Input: dimensioned drawing with shaded views. Units: mm. Origin: part minimum x, y, z. A direction names the side the tool comes from. Coordinates: 2 decimals unless noted, no trailing zeros. Write each loop counter-clockwise with the first axis right and the second up, starting at its lowest first coordinate (ties: lowest second). Pieces come first, ordered by that corner, then holes. Notation, with made-up numbers: (15.25, 8.5) -> (37.25, 8.5) arc R26 ccw to (37.25, 26.5) -> close; hole circle Ø5 at (-17, 63.5). An arc over 180 degrees is marked (long way). One line per item, written item: value. Start each with the question number.
1. Section query A-A, the plane y = 12. Output: boundary loops of the cut face in (x, z), and give its area (3 significant figures).
2. Access query for the marked faces 4 and 5. Directions: +Z, -Z, +X, -X, +Y, -Y. A direction counts if a zero-diameter tool reaches every point of the face in a straight line with its end or side. Return the directions, or none.
3. First-contact query: P1, Ø1.5, axis at x = 19, z = 3.5, coming from the +Y side; P2, Ø1, axis at y = 21, z = 3, coming from the -X side; P3, Ø7, axis at x = 12, y = 12, coming from the -Z side; P4, Ø8, axis at x = 11, y = 14.5, coming from the +Z side. Flat tips, straight axial feed; report the tip coordinate or a pass-through.
4. Mould query, pull axis X, two halves, no side actions, for the marked faces 1, 2 and 3. Classes: released by +X, released by -X, zero draft, split by the parting line, or undercut.
5. Section query D-D, the plane z = 4.6. Output: boundary loops of the cut face in (x, y).
6. Section query C-C, the plane z = 0.9. Output: boundary loops of the cut face in (x, y), and give its area (3 significant figures).
7. Line query: line 1 (Y direction, x = 12, z = 2.15); line 2 (Y direction, x = 12, z = 4.6); line 3 (Z direction, x = 17.5, y = 8.75). Output: solid intervals per line, ascending.
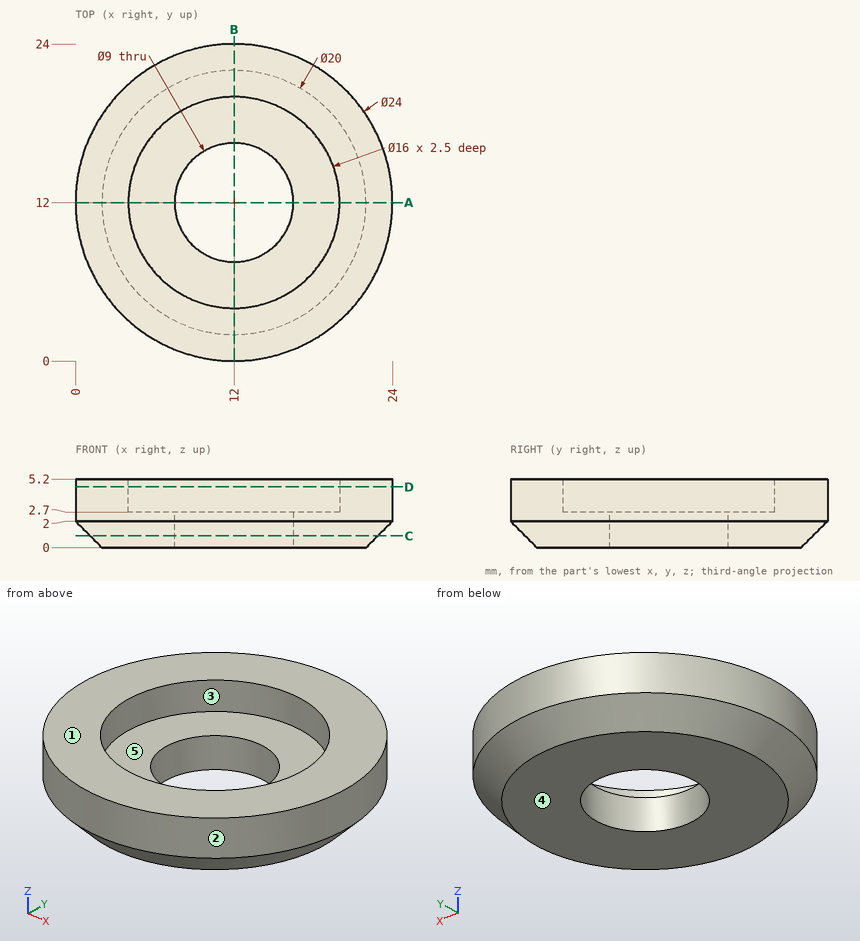
Computed values:
1. outline: (0, 2) -> (2, 0) -> (7.5, 0) -> (7.5, 2.7) -> (4, 2.7) -> (4, 5.2) -> (0, 5.2) -> close; (16.5, 0) -> (22, 0) -> (24, 2) -> (24, 5.2) -> (20, 5.2) -> (20, 2.7) -> (16.5, 2.7) -> close
1. area: 56.5 mm²
2. face 4: -Z, +X, -X, +Y, -Y
2. face 5: +Z
3. P1: stops at y = 22.24
3. P2: stops at x = 3.53
3. P3: passes through
3. P4: stops at z = 2.7
4. face 1: zero draft
4. face 2: split by the parting line
4. face 3: undercut
5. outline: circle Ø24 at (12, 12); hole circle Ø16 at (12, 12)
6. outline: circle Ø21.8 at (12, 12); hole circle Ø9 at (12, 12)
6. area: 310 mm²
7. line 1: y = 0 to 7.5, 16.5 to 24
7. line 2: y = 0 to 4, 20 to 24
7. line 3: z = 0 to 2.7
